Part print with two shaded views. Sizes in mm from the minimum x, y, z corner. Give positions to 0.01 mm unless a question says otherwise; leave off trailing zeros. Order: outer loops, then holes, each group sorted by start corner. A loop starts at its lowest first (then second) coordinate and runs counter-clockwise, first axis right, second up.
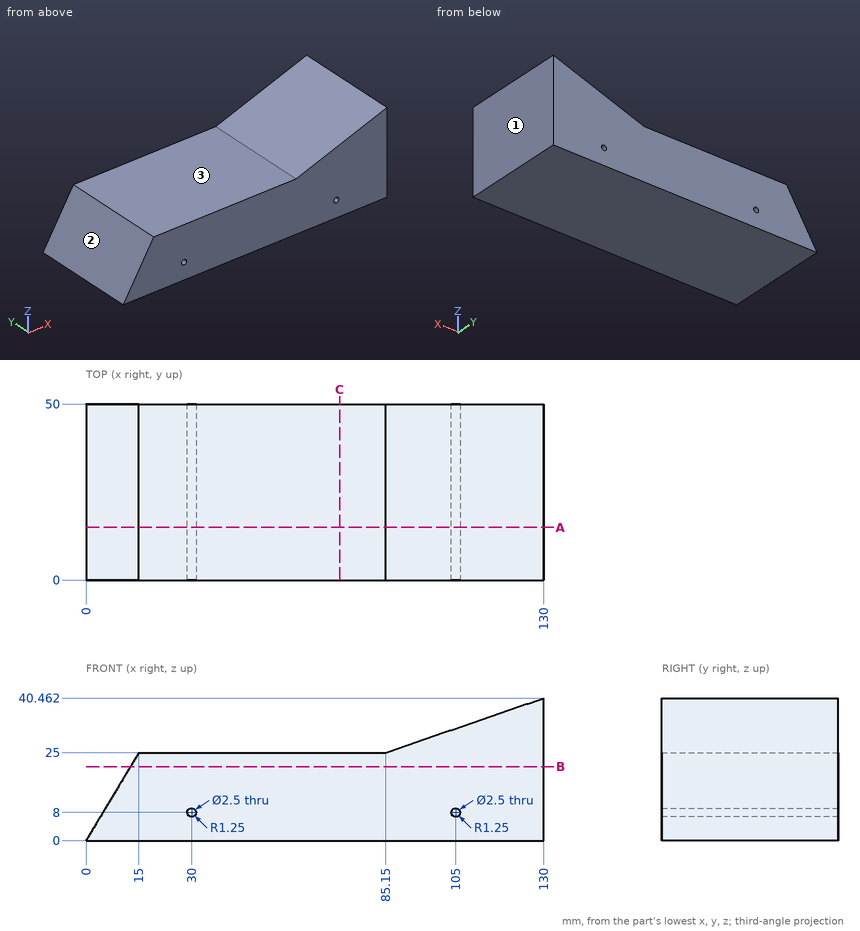
1. Saw through at B-B on z = 21. Give the cut face in (x, y), plus the area to 3 significant figures.
2. Saw through at A-A on y = 15. Give the cut face in (x, z).
3. Wall check: line 1 (Z direction, x = 30, y = 14); line 2 (X direction, y = 22, z = 8); line 3 (Z direction, x = 105, y = 24). Give the ranges that are in metal, low to high.
4. Pin check, flat tips, straight feed: P1, Ø1, axis at y = 23, z = 23, coming from the -X side; P2, Ø3, axis at x = 60, y = 13.5, coming from the +Z side. Stop position of each tip, or through.
5. Saw through at C-C on x = 72. Give the cut face in (y, z).
6. Mould opens along X. For the marked faces 1, 2 and 3 say: released by +X, released by -X, zero draft, split by the parting line, or undercut.
Reported:
1. outline: (12.6, 0) - (130, 0) - (130, 50) - (12.6, 50) - close
1. area: 5,870 mm2
2. outline: (0, 0) - (130, 0) - (130, 40.46) - (85.15, 25) - (15, 25) - close; hole (30, 6.75) arc R1.25 ccw to (31.25, 8) arc R1.25 ccw (long way) to start; hole (105, 6.75) arc R1.25 ccw to (106.25, 8) arc R1.25 ccw (long way) to start
3. line 1: z = 0 to 6.75, 9.25 to 25
3. line 2: x = 4.8 to 28.75, 31.25 to 103.75, 106.25 to 130
3. line 3: z = 0 to 6.75, 9.25 to 31.84
4. P1: stops at x = 13.5
4. P2: stops at z = 25
5. outline: (0, 0) - (50, 0) - (50, 25) - (0, 25) - close
6. face 1: released by +X
6. face 2: released by -X
6. face 3: zero draft
